from build123d import *

# Parameters (mm, degrees)
SKETCH001_R                    = 9
EXTRUDE001_DEPTH               = 10
SKETCH_AS_DRAWN_W              = 73
SKETCH_AS_DRAWN_H              = 27
EXTRUDE_DEPTH                  = 10
EXTRUDE_ONTO_SKETCH_ROLL_ANGLE = 90
BOX_W                          = 145
BOX_H                          = 146
BOX_DEPTH                      = 57
BOX001_W                       = 150
BOX001_H                       = 150
BOX001_DEPTH                   = 60
CHAMFER001_SIZE                = 1


with BuildPart() as obj1:
    # Sketch001 → Extrude001 (new body)
    with BuildSketch(Plane.YZ.offset(150)):
        with Locations((129.311707, 12.728212)):
            Circle(SKETCH001_R)
    extrude(amount=EXTRUDE001_DEPTH)


with BuildPart() as obj1_1:
    # Extrude001 placement: moved
    add(obj1.part.moved(Location((-6, 1, 5))))


with BuildPart() as fusion:
    # Sketch as drawn → Extrude (new)
    with BuildSketch(Plane.XY):
        with Locations((101.75337, 31.497138)):
            Rectangle(SKETCH_AS_DRAWN_W, SKETCH_AS_DRAWN_H)
    extrude(amount=EXTRUDE_DEPTH)


with BuildPart() as fusion_1:
    # Extrude onto Sketch roll: moved
    add(fusion.part.rotate(Axis((0, 0, 0), (1, 0, 0)), EXTRUDE_ONTO_SKETCH_ROLL_ANGLE))


with BuildPart() as fusion_2:
    # Extrude onto Sketch placement: moved
    add(fusion_1.part)


with BuildPart() as fusion_3:
    # Extrude placement: moved
    add(fusion_2.part.moved(Location((0, 6, 0))))

    # Fusion: union obj1
    add(obj1_1.part)


with BuildPart() as cubo:
    # Box → Box (new body)
    with BuildSketch(Plane(origin=(3, 2, 5), x_dir=(1, 0, 0), z_dir=(0, 0, 1))):
        with Locations((72.5, 73)):
            Rectangle(BOX_W, BOX_H)
    extrude(amount=BOX_DEPTH)


with BuildPart() as basecaja:
    # Box001 → Box001 (new body)
    with BuildSketch(Plane.XY):
        with Locations((75, 75)):
            Rectangle(BOX001_W, BOX001_H)
    extrude(amount=BOX001_DEPTH)

    # Cut: cut Cubo
    add(cubo.part, mode=Mode.SUBTRACT)

    # Cut001: cut Fusion
    add(fusion_3.part, mode=Mode.SUBTRACT)

    # Chamfer001
    chamfer001_edges = [basecaja.edges().sort_by_distance(p)[0] for p in [
        (75.5, 2, 60),
        (148, 75, 60),
        (75.5, 148, 60),
        (3, 75, 60),
    ]]
    chamfer(chamfer001_edges, length=CHAMFER001_SIZE)


solid = basecaja.part
Geometry: final body of the model. Coordinates: model frame, mm. A direction names the side the tool comes from. Round coordinates to 2 decimals unless told otherwise and drop trailing zeros. Loops run counter-clockwise (first coordinate to the right, second up) from the corner with the lowest first, then second, coordinate; pieces in that order, holes last. Notation, with made-up numbers: M 65,86 L 110,86 A33 cw 110,122 Z; hole C -39,13 d1. An arc over 180 degrees is marked long. Put each result on its own line as item: value. Start each with the question number.
(1) Section query C-C (y = 132). Return loops of the section in (x, z), then the cut area to 3 significant figures.
(2) Section query B-B (z = 55.5). Return loops of the section in (x, y), then the cut area to 3 significant figures.
(3) Section query A-A (x = 125.5). Return loops of the section in (y, z).
(4) Material intervals for line 1 along X through (y, z) = (115.5, 25.5); line 2 along Y through (x, z) = (76, 48.5); line 3 along Y through (x, z) = (105.5, 32), sorted ascending. Write a range as [from, to].
(5) Draft query along Z for faces 3 (the face through (74, 76, 0)), 4 (the face through (74, 76, 5)), 5 (the face through (0, 74, 30)), 6 (the face through (148.99, 121.32, 18.12)). Return one class per face: +Z half, -Z half, draft (parallel to the pull), parting line (faces both ways), or undercut.
(6) Section query D-D (y = 51). Return loops of the section in (x, z).
(7) Set-up query: faces 1 (the face through (150, 74, 30)), 2 (the face through (3, 74, 32)). Return all of +Z, -Z, +X, -X, +Y, -Y with unobstructed straight access to the full face (end or side cutting, diameter ignored); none if empty.
(8) Contact query for flat-ended pins moving along their axis: pin 1 Ø1 at (y, z) = (1.5, 33.5) entering from -X; pin 2 Ø4 at (x, z) = (127, 21) entering from -Y. Output: stop coordinate, or through.
Findings below:
1. outline: M 0,0 L 150,0 L 150,8.89 L 148,8.89 L 148,5 L 3,5 L 3,59 L 2,60 L 0,60 Z; M 148,26.57 L 150,26.57 L 150,60 L 149,60 L 148,59 Z
1. area: 989 mm2
2. outline: M 0,0 L 150,0 L 150,150 L 0,150 Z; hole M 3,2 L 148,2 L 148,148 L 3,148 Z
2. area: 1,330 mm2
3. outline: M 0,0 L 150,0 L 150,60 L 149,60 L 148,59 L 148,5 L 2,5 L 2,18 L 0,18 Z; M 0,45 L 2,45 L 2,59 L 1,60 L 0,60 Z
4. line 1: x = [0, 3], [148, 150]
4. line 2: y = [0, 2], [148, 150]
4. line 3: y = [148, 150]
5. face 3: -Z half
5. face 4: +Z half
5. face 5: draft
5. face 6: undercut
6. outline: M 0,0 L 150,0 L 150,60 L 149,60 L 148,59 L 148,5 L 3,5 L 3,59 L 2,60 L 0,60 Z
7. face 1: +Z, -Z, +X, +Y, -Y
7. face 2: +Z
8. pin 1: stops at x = 0
8. pin 2: stops at y = 148
